Read the model definition and answer for the solid it produces. Units are mm, in the model's axes. A direction names the side the tool comes from. Coordinates: 2 decimals unless noted, no trailing zeros. Loops run counter-clockwise (first coordinate to the right, second up) from the corner with the lowest first, then second, coordinate; pieces in that order, holes last.
Autodesk Inventor part; units mm, degrees
ref_plane "YZ Plane" through (0, 0, 0) normal (1, 0, 0) x (0, 1, 0)
ref_plane "XZ Plane" through (0, 0, 0) normal (0, 1, 0) x (-1, 0, 0)
ref_plane "XY Plane" through (0, 0, 0) normal (0, 0, 1) x (1, 0, 0)
sketch "Sketch1" plane through (0, 0, 0) normal (0, 1, 0) x (-1, 0, 0)
  circle A0 centre (0, 0) radius 254
  circle A1 centre (0, 0) radius 279.4
  line L0 (0, 279.4) -> (0, -279.4)
  line L1 (-279.4, 0) -> (279.4, 0)
  line L2 (197.5656, -197.5656) -> (-197.5656, 197.5656)
  line L3 (197.5656, 197.5656) -> (-197.5656, -197.5656)
  line L4 (206.5459, -188.5854) -> (-188.5854, 206.5459)
  line L5 (188.5854, -206.5459) -> (-206.5459, 188.5854)
  line L6 (188.5854, 206.5459) -> (-206.5459, -188.5854)
  line L7 (206.5459, 188.5854) -> (-188.5854, -206.5459)
  circle A2 centre (0, 0) radius 152.4
  circle A3 centre (0, 0) radius 101.6
  circle A4 centre (0, 0) radius 88.9
  circle A5 centre (0, 0) radius 139.7
  circle A6 centre (146.05, 0) radius 3.175
  circle A7 centre (73.025, 126.483) radius 3.175
  circle A8 centre (-73.025, 126.483) radius 3.175
  circle A9 centre (-146.05, 0) radius 3.175
  circle A10 centre (-73.025, -126.483) radius 3.175
  circle A11 centre (73.025, -126.483) radius 3.175
  circle A12 centre (95.25, 0) radius 3.175
  circle A13 centre (47.625, 82.4889) radius 3.175
  circle A14 centre (-47.625, 82.4889) radius 3.175
  circle A15 centre (-95.25, 0) radius 3.175
  circle A16 centre (-47.625, -82.4889) radius 3.175
  circle A17 centre (47.625, -82.4889) radius 3.175
  circle A18 centre (0, 0) radius 284.48
  dimension "d0" = 508
  dimension "d1" = 25.4
  dimension "d2" = 45
  dimension "d3" = 0
  dimension "d4" = 0
  dimension "d5" = 45
  dimension "d6" = 12.7
  dimension "d7" = 12.7
  dimension "d8" = 12.7
  dimension "d9" = 12.7
  dimension "d10" = 304.8
  dimension "d11" = 203.2
  dimension "d12" = 177.8
  dimension "d13" = 12.7
  dimension "d14" = 6.35
  dimension "d15" = 146.05
  dimension "d18" = 360
  dimension "d20" = 6.35
  dimension "d21" = 95.25
  dimension "d24" = 360
  dimension "d26" = 5.08
extrude "Extrusion1" add sketch "Sketch1" along normal blind 5.08 contours L1 A2 L7 A0 | L1 A1 L4 A0 | A0 L4 A2 L1 | A0 L7 A1 L1 | L7 A2 L3 A0 | A0 L3 A1 L7 | L4 A1 L2 A0 | A0 L2 A2 L4 | A2 L4 A5 L1 A6 | L1 A6 A5 L7 A2 | L3 A2 L6 A0 | A0 L6 A1 L3 | L7 A5 L3 A2 | L2 A1 L5 A0 | A0 L5 A2 L2 | A2 L2 A5 L4 | A6 L1 | L1 A6 | L6 A2 L0 A0 | A0 L0 A1 L6 | L3 A5 L6 A2 | A5 L1 A3 L7 | L7 A3 L3 A5 | L5 A1 L0 A0 | A0 L0 A2 L5 | A2 L5 A5 L2 | A5 L2 A3 L4 | L4 A3 L1 A5 | L0 A2 L4 A0 | A0 L4 A1 L0 | L6 A5 L0 A2 | L3 A3 L6 A5 | A3 L1 A12 A4 L7 | L7 A4 L3 A3 | L0 A1 L7 A0 | A0 L7 A2 L0 | A2 L0 A5 L5 | A5 L5 A3 L2 | A3 L2 A4 L4 | L4 A4 L1 A12 A3 | L4 A2 L2 A0 | A0 L2 A1 L4 | L0 A5 L4 A2 | L6 A3 L0 A5 | L3 A4 L6 A3 | A4 L1 L7 | L7 L4 L3 A4 | L7 A1 L3 A0 | A0 L3 A2 L7 | A2 L7 A5 L0 | A5 L0 A3 L5 | A3 L5 A4 L2 | A4 L2 L7 L4 | L4 L1 A4 | L2 A2 L5 A0 | A0 L5 A1 L2 | L4 A5 L2 A2 | L0 A3 L4 A5 | L6 A4 L0 A3 | L3 L4 L6 A4 | L7 L2 L1 | L1 L3 L4 | L3 A1 L6 A0 | A0 L6 A2 L3 | A2 L3 A5 L7 | A5 L7 A3 L0 | A3 L0 A4 L5 | A4 L5 L7 L2 | L5 A2 L1 A0 | A0 L1 A1 L5 | L2 A5 L5 A2 | L4 A3 L2 A5 | L0 A4 L4 A3 | L6 L0 A4 | L3 L0 L4 | L2 L6 L0 | L2 L7 L0 | L3 L5 L1 | L1 L6 L2 | L0 L5 L3 | L6 A1 L1 A0 | A0 L1 A2 L6 | A2 L6 A5 L3 | A5 L3 A3 L7 | A3 L7 A4 L0 | A4 L0 L5 | L5 A5 L1 A9 A2 | L2 A3 L5 A5 | L4 A4 L2 A3 | L0 L4 A4 | L6 L2 A4 L4 | L7 A4 L3 L5 | L0 A4 L7 | L6 A4 L1 | L1 A4 L5 | L5 A4 L2 L6 | L5 L3 A4 L6 | A2 L1 A9 A5 L6 | A5 L6 A3 L3 | A3 L3 A4 L7 | L5 A3 L1 A5 | L2 A4 L5 A3 | A4 L6 A3 L1 A15 | L1 A15 A3 L5 A4 | A4 L3 A3 L6 | A5 L1 A3 L6 | A9 L1 | L1 A9 | A7 | A8 | A10 | A11 | A18
extrude "Extrusion2" add sketch "Sketch1" against normal blind 25.4 contours A18
properties part number "Lazy suzan Top piece"
Q1. Determine the mould class of faces 1 (the face through (-209, -25.4, -188)), 2 (the face through (221.722, -12.522, -170.011)), 3 (the face through (61.67, -9.947, -277.715)) for opening direction X: +X half, -X half, draft (parallel to the pull), parting line (faces both ways), or undercut.
Findings below:
face 1: draft
face 2: undercut
face 3: parting line
Q2. Which of the six approach directions +Z, -Z, +X, -X, +Y, -Y give full straight-line access (tool end or side, diameter ignored) to faces 4 (the face through (4, 5.08, 4)), 5 (the face through (4, 0, 4))?
Findings below:
face 4: +Z, -Z, +X, -X, +Y
face 5: -Y
Q3. A cutting plane is placed at C-C (z = 236). Give the vertices of the cut face in (x, y), then the cut area to 3 significant figures.
Findings below:
outline: (-158.85, -25.4) - (-149.56, -25.4) - (-149.56, 0) - (149.56, 0) - (149.56, -25.4) - (158.85, -25.4) - (158.85, 5.08) - (-158.85, 5.08) - close
area: 2,090 mm2
Q4. A cutting plane is placed at B-B (y = -20). Give the vertices of the cut face in (x, z), then the cut area to 3 significant figures.
Findings below:
outline: circle Ø568.96 at (0, 0); hole circle Ø558.8 at (0, 0)
area: 9,000 mm2
Q5. Flat-ended cylindrical pins translate along their axes: pin 1 Ø1.5 at (x, z) = (45, -35.5) entering from -Y; pin 2 Ø10 at (x, y) = (47.5, 0) entering from +Z; pin 3 Ø1 at (x, y) = (31, 0) entering from +Z; pin 4 Ø4 at (x, z) = (47.62, -82.49) entering from -Y. Find the tip coordinate at first contact, or state that the pin passes through.
Findings below:
pin 1: stops at y = 0
pin 2: stops at z = 281.29
pin 3: stops at z = 282.84
pin 4: passes through
Q6. Straight lines are drawn through the part: probe 1 along Z at (x, y) = (-95.25, 3.7) (3 decimals); probe 2 along Z at (x, y) = (173.5, -14.5); probe 3 along X at (y, z) = (-8, 175.5). For each, find the intervals that lie inside material, in ascending order.
Findings below:
probe 1: z = -268.06 to -3.175, 3.175 to 268.06
probe 2: z = -225.45 to -219, 219 to 225.45
probe 3: x = -223.89 to -217.4, 217.4 to 223.89
Q7. A cutting plane is placed at A-A (x = 0). Give the vertices of the cut face in (y, z).
Findings below:
outline: (-25.4, -284.48) - (5.08, -284.48) - (5.08, 284.48) - (-25.4, 284.48) - (-25.4, 279.4) - (0, 279.4) - (0, -279.4) - (-25.4, -279.4) - close
